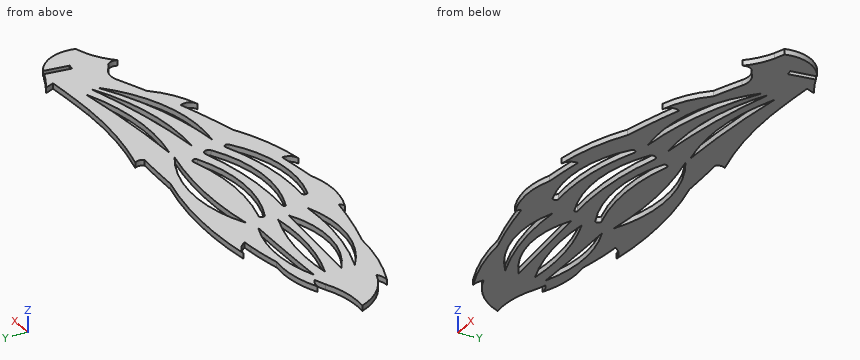
```python
from build123d import *

# Parameters (mm, degrees)
BOSS_EXTRUDE1_DEPTH = 1.524


with BuildPart() as part:
    # Model → Boss-Extrude1 (new body)
    with BuildSketch(Plane.XY):
        with BuildLine():
            Line((125.457442265, 29.854729058), (124.36118777, 22.768051361))
            Line((124.36118777, 22.768051361), (125.867274198, 22.535071382))
            Line((125.867274198, 22.535071382), (126.914488667, 29.304732487))
            ThreePointArc((126.914488667, 29.304732487), (131.596034511, 24.191259053), (132.080813549, 17.27537362))
            Line((132.080813549, 17.27537362), (129.201538518, 16.231235276))
            ThreePointArc((129.201538518, 16.231235276), (125.494314224, 14.202109959), (122.342593367, 11.386525267))
            ThreePointArc((122.342593367, 11.386525267), (122.521547644, 13.015286897), (121.637755911, 14.395069943))
            ThreePointArc((121.637755911, 14.395069943), (120.558535261, 14.894839146), (119.655012959, 15.668230327))
            ThreePointArc((119.655012959, 15.668230327), (116.945656671, 16.627230011), (114.111435919, 16.150276533))
            ThreePointArc((114.111435919, 16.150276533), (110.130348083, 14.492411945), (106.116427247, 12.915701804))
            ThreePointArc((106.116427247, 12.915701804), (100.871077069, 8.483544727), (94.612309809, 5.65767367))
            ThreePointArc((94.612309809, 5.65767367), (96.234412345, 7.167311858), (96.088279041, 9.378390589))
            ThreePointArc((96.088279041, 9.378390589), (87.959563224, 6.916430033), (79.738932416, 4.781365698))
            ThreePointArc((79.738932416, 4.781365698), (70.087015382, 0.573629162), (59.825334355, -1.784855875))
            ThreePointArc((59.825334355, -1.784855875), (61.625546567, -0.674388225), (62.177186804, 1.367570505))
            ThreePointArc((62.177186804, 1.367570505), (56.69945513, 0.613180121), (51.20394484, 0.001611808))
            ThreePointArc((51.20394484, 0.001611808), (42.783253785, -1.45847583), (34.430253575, 0.349086412))
            ThreePointArc((34.430253575, 0.349086412), (35.242407465, 0.582998344), (35.696308866, 1.295937508))
            ThreePointArc((35.696308866, 1.295937508), (26.899874012, 2.912690878), (18.24226034, 5.156991018))
            ThreePointArc((18.24226034, 5.156991018), (8.327270493, 6.613476825), (-1.186477097, 9.762600728))
            ThreePointArc((-1.186477097, 9.762600728), (0.567723509, 9.933888345), (2.129376981, 10.751077214))
            ThreePointArc((2.129376981, 10.751077214), (-4.564424076, 14.67509235), (-8.866303828, 21.132545253))
            ThreePointArc((-8.866303828, 21.132545253), (-2.028267146, 21.342243043), (4.458921798, 23.51459164))
            ThreePointArc((4.458921798, 23.51459164), (5.978589155, 24.100559155), (7.508094135, 24.660346004))
            ThreePointArc((7.508094135, 24.660346004), (6.073839254, 25.435989759), (4.458921798, 25.661271599))
            ThreePointArc((4.458921798, 25.661271599), (11.846812063, 27.976344953), (19.588212991, 28.082169784))
            ThreePointArc((19.588212991, 28.082169784), (24.23969735, 28.951914388), (28.92877134, 29.588583491))
            ThreePointArc((28.92877134, 29.588583491), (30.250891965, 29.696247396), (31.57341018, 29.798912074))
            ThreePointArc((31.57341018, 29.798912074), (29.710039, 31.839896858), (27.095456614, 32.73529062))
            ThreePointArc((27.095456614, 32.73529062), (46.017315853, 33.521760077), (64.749650783, 30.73699449))
            ThreePointArc((64.749650783, 30.73699449), (71.265909378, 30.552300799), (77.77761193, 30.246575893))
            ThreePointArc((77.77761193, 30.246575893), (78.240878226, 31.474299031), (77.877808016, 32.73529062))
            ThreePointArc((77.877808016, 32.73529062), (91.368554355, 30.154894712), (105.083859187, 29.413886469))
            ThreePointArc((105.083859187, 29.413886469), (112.860951548, 29.721873992), (120.624125013, 30.279690879))
            ThreePointArc((120.624125013, 30.279690879), (120.101426826, 31.522338532), (119.655012959, 32.794384617))
            ThreePointArc((119.655012959, 32.794384617), (122.492136598, 31.198051004), (125.457442265, 29.854729058))
        make_face()
        with BuildLine():
            ThreePointArc((113.344379689, 22.19615093), (96.963122218, 12.553503985), (77.990394499, 11.386525267))
            ThreePointArc((77.990394499, 11.386525267), (96.271224533, 14.816426058), (113.344379689, 22.19615093))
        make_face(mode=Mode.SUBTRACT)
        with BuildLine():
            ThreePointArc((113.344379689, 23.82080051), (96.187450512, 17.719248724), (77.990394499, 17.043744891))
            ThreePointArc((77.990394499, 17.043744891), (95.848162694, 19.489217449), (113.344379689, 23.82080051))
        make_face(mode=Mode.SUBTRACT)
        with BuildLine():
            ThreePointArc((112.010038699, 26.273742515), (95.04541072, 22.055495603), (77.613248587, 23.363904105))
            ThreePointArc((77.613248587, 23.363904105), (94.856261251, 24.29140484), (112.010038699, 26.273742515))
        make_face(mode=Mode.SUBTRACT)
        with BuildLine():
            ThreePointArc((73.920433764, 9.144198092), (59.762067232, 3.425519676), (44.552717894, 4.781365698))
            ThreePointArc((44.552717894, 4.781365698), (44.052345371, 5.659967485), (44.86760609, 6.258017419))
            ThreePointArc((44.86760609, 6.258017419), (59.284947166, 6.637177896), (73.189879005, 10.465540071))
            ThreePointArc((73.189879005, 10.465540071), (74.143785851, 10.130315533), (73.920433764, 9.144198092))
        make_face(mode=Mode.SUBTRACT)
        with BuildLine():
            ThreePointArc((73.7171882, 14.19085222), (74.195068041, 15.63804442), (72.809895852, 16.27367986))
            ThreePointArc((72.809895852, 16.27367986), (57.603683966, 13.161162203), (42.082533848, 13.058472776))
            ThreePointArc((42.082533848, 13.058472776), (41.678568271, 12.772614258), (41.897709615, 12.328902245))
            ThreePointArc((41.897709615, 12.328902245), (58.027223609, 9.504074716), (73.7171882, 14.19085222))
        make_face(mode=Mode.SUBTRACT)
        with BuildLine():
            ThreePointArc((71.615953494, 19.263251529), (72.005249, 20.227653753), (71.069824737, 20.682190977))
            ThreePointArc((71.069824737, 20.682190977), (55.942470801, 18.367444511), (40.793050931, 20.533077418))
            ThreePointArc((40.793050931, 20.533077418), (39.862149142, 20.069348511), (40.260924923, 19.10882755))
            ThreePointArc((40.260924923, 19.10882755), (55.955346454, 15.753106638), (71.615953494, 19.263251529))
        make_face(mode=Mode.SUBTRACT)
        with BuildLine():
            ThreePointArc((75.249897816, 23.419828185), (57.358073705, 25.777828917), (39.34157015, 24.737090166))
            ThreePointArc((39.34157015, 24.737090166), (57.468271047, 28.781788902), (75.249897816, 23.419828185))
        make_face(mode=Mode.SUBTRACT)
        with BuildLine():
            ThreePointArc((38.218093055, 8.509361046), (23.282181122, 9.069608784), (8.79939997, 12.763440518))
            ThreePointArc((8.79939997, 12.763440518), (22.937130999, 6.683446576), (38.218093055, 8.509361046))
        make_face(mode=Mode.SUBTRACT)
        with BuildLine():
            ThreePointArc((37.366333435, 14.19085222), (23.274365612, 15.219049254), (9.184351398, 16.27367986))
            ThreePointArc((9.184351398, 16.27367986), (22.976923316, 11.194465897), (37.366333435, 14.19085222))
        make_face(mode=Mode.SUBTRACT)
        with BuildLine():
            ThreePointArc((36.84813704, 17.413649418), (23.030567399, 17.299167045), (9.596276919, 20.533077418))
            ThreePointArc((9.596276919, 20.533077418), (23.40846607, 20.600554903), (36.84813704, 17.413649418))
        make_face(mode=Mode.SUBTRACT)
        with BuildLine():
            ThreePointArc((35.94161169, 23.51459164), (22.768944305, 23.628526918), (9.596276919, 23.51459164))
            ThreePointArc((9.596276919, 23.51459164), (22.768944305, 26.146058656), (35.94161169, 23.51459164))
        make_face(mode=Mode.SUBTRACT)
    extrude(amount=BOSS_EXTRUDE1_DEPTH)


solid = part.part
```
CAD build for the part. Positions are in the model's coordinates, mm. Round coordinates to 2 decimals unless told otherwise and drop trailing zeros. Write each loop counter-clockwise with the first axis right and the second up, starting at its lowest first coordinate (ties: lowest second). Pieces come first, ordered by that corner, then holes. Notation, with made-up numbers: (69.5, 68.25) - (88.5, 68.25) arc R17 ccw to (88.5, 91.25) - close; hole circle Ø6 at (80, -2.5). An arc over 180 degrees is marked (long way). Write item = value, one per line. Start each with the question number.
Q1. Band-saw the part on D-D (x = 117). Give the cut face in (y, z), then the cut area to 3 significant figures.
Q2. Band-saw the part on B-B (x = 90.5). Give the cut face in (y, z), then the cut area to 3 significant figures.
Q3. Band-saw the part on C-C (z = 0.5). Count the separate pieces of the cut face and the enclosed holes in it, then the cut area to 3 significant figures.
Q4. Band-saw the part on A-A (x = 25.5). Give the cut face in (y, z).
Q5. Probe L1, parallel to Y at x = 20.5, z = 0.45; L2, parallel to Y at x = 94, z = 1.05; L3, parallel to Y at x = 93.5, z = 0.7. List the from-to ranges inside material, lowest first. Write a range as from..to.
Answers below:
q1.outline = (16.62, 0) - (29.99, 0) - (29.99, 1.52) - (16.62, 1.52) - close
q1.area = 20.4 mm2
q2.outline = (7.65, 0) - (11.14, 0) - (11.14, 1.52) - (7.65, 1.52) - close; (13.27, 0) - (16.91, 0) - (16.91, 1.52) - (13.27, 1.52) - close; (18.55, 0) - (21.86, 0) - (21.86, 1.52) - (18.55, 1.52) - close; (23.96, 0) - (30.26, 0) - (30.26, 1.52) - (23.96, 1.52) - close
q2.area = 25.5 mm2
q3.separate_pieces = 1
q3.enclosed_holes = 11
q3.area = 2,540 mm2
q4.outline = (3.23, 0) - (6.43, 0) - (6.43, 1.52) - (3.23, 1.52) - close; (8.78, 0) - (11.13, 0) - (11.13, 1.52) - (8.78, 1.52) - close; (15.05, 0) - (17.07, 0) - (17.07, 1.52) - (15.05, 1.52) - close; (20.32, 0) - (23.62, 0) - (23.62, 1.52) - (20.32, 1.52) - close; (26.04, 0) - (29.15, 0) - (29.15, 1.52) - (26.04, 1.52) - close
q5.L1 = 4.51..7.14, 9.53..11.49, 15.42..17.65, 20.86..23.63, 26.07..28.27
q5.L2 = 8.71..11.77, 14.16..17.34, 19.15..21.98, 24.22..29.87
q5.L3 = 8.56..11.66, 14.02..17.27, 19.06..21.95, 24.18..29.92
